Here's how the part is built. I have some questions about the finished solid (model axes, mm). A direction names the side the tool comes from. Coordinates: 2 decimals unless noted, no trailing zeros. Write each loop counter-clockwise with the first axis right and the second up, starting at its lowest first coordinate (ties: lowest second). Pieces come first, ordered by that corner, then holes.
Item 1: I want a section at C-C (x = 35.55). Please give me the cut outline in (y, z), and give its area (3 significant figures).
Item 2: I'm going to push flat-ended pins straight in: P1, Ø1.5, axis at x = 32, z = 6, coming from the -Y side; P2, Ø1.9, axis at x = 3.5, y = 3.5, coming from the -Z side; P3, Ø2, axis at y = -0.5, z = 2.5, coming from the -X side; P4, Ø3, axis at x = 24, y = -0.5, coming from the +Z side. Where does each tip first touch, or does it pass through?
Item 3: I want a section at D-D (y = -6.5). Please give me the cut outline in (x, z).
Item 4: I want a section at B-B (y = 10.65). Please give me the cut outline in (x, z).
Item 5: Please list where these lines run through material, in increasing order: line 1 (Y direction, x = 42.2, z = 0.8); line 2 (Y direction, x = 3.5, z = 1); line 3 (Z direction, x = 21, y = 5.5).
Item 6: I want a section at A-A (z = 2.5). Please give me the cut outline in (x, y).
Item 7: For faces 1 (the face through (25.85, 0, 2)), 2 (the face through (10, 11, 14.5)), 3 (the face through (24.35, -4.7, 2.48)), which set-ups out of +Z, -Z, +X, -X, +Y, -Y let a thin tool reach every point of the face, with its end or its side?
Autodesk Inventor part; units mm, degrees
ref_plane "YZ Plane" through (0, 0, 0) normal (1, 0, 0) x (0, 1, 0)
ref_plane "XZ Plane" through (0, 0, 0) normal (0, 1, 0) x (-1, 0, 0)
ref_plane "XY Plane" through (0, 0, 0) normal (0, 0, 1) x (1, 0, 0)
sketch "スケッチ1" plane through (0, 0, 0) normal (0, 0, 1) x (1, 0, 0)
  line L0 (0, 0) -> (45.7, 0)
  line L1 (45.7, 0) -> (45.7, 21.3)
  line L2 (45.7, 21.3) -> (0, 21.3)
  line L3 (0, 21.3) -> (0, 0)
  line L4 (45.7, 21.3) -> (42.2, 21.3) construction
  line L5 (42.2, 21.3) -> (42.2, 17.8) construction
  line L6 (42.2, 17.8) -> (45.7, 17.8) construction
  line L7 (45.7, 17.8) -> (45.7, 21.3) construction
  line L8 (0, 0) -> (3.5, 0) construction
  line L9 (3.5, 0) -> (3.5, 3.5) construction
  line L10 (3.5, 3.5) -> (0, 3.5) construction
  line L11 (0, 3.5) -> (0, 0) construction
  circle A0 centre (3.5, 3.5) radius 1.55
  circle A1 centre (42.2, 17.8) radius 1.55
  dimension "d0" = 45.7
  dimension "d1" = 21.3
  dimension "d2" = 3.5
  dimension "d3" = 3.5
  dimension "d4" = 3.5
  dimension "d5" = 3.5
  dimension "d6" = 3.1
  dimension "d7" = 3.1
extrude "押し出し1" add sketch "スケッチ1" along normal blind 1.5
sketch "スケッチ2" plane through (0, 0, 1.5) normal (0, 0, 1) x (1, 0, 0)
  line L0 (0, 21.3) -> (0, 0) construction
  line L1 (0, 10.65) -> (2, 10.65) construction
  line L2 (2, 10.65) -> (18.3, 10.65) construction
  line L3 (18.3, 10.65) -> (27.4, 10.65) construction
  line L4 (27.4, 10.65) -> (43.7, 10.65) construction
  line L5 (43.7, 10.65) -> (45.7, 10.65) construction
  circle A0 centre (10.15, 10.65) radius 8
  circle A1 centre (35.55, 10.65) radius 8
  dimension "d10" = 2
  dimension "d11" = 16.3
  dimension "d12" = 9.1
  dimension "d13" = 16.3
  dimension "d14" = 2
  dimension "d15" = 16
  dimension "d16" = 16
extrude "押し出し2" add sketch "スケッチ2" along normal blind 14
sketch "スケッチ3" plane through (10.15, 10.65, 15.5) normal (0, 0, 1) x (1, 0, 0)
  circle A0 centre (0, 0) radius 6.5
  circle A1 centre (25.4, 0) radius 8
  circle A2 centre (25.4, 0) radius 6.5
  point P0 (-10.15, -10.65)
  dimension "d19" = 13
  dimension "d20" = 13
extrude "押し出し3" cut sketch "スケッチ3" against normal blind 1 contours A0 | A2
sketch "スケッチ4" plane through (0, 0, 1.5) normal (0, 0, 1) x (1, 0, 0)
  line L0 (19.85, -1.25) -> (25.85, -1.25)
  line L1 (25.85, -1.25) -> (25.85, 1.25)
  line L2 (25.85, 1.25) -> (19.85, 1.25)
  line L3 (19.85, 1.25) -> (19.85, -1.25)
  line L4 (0, 0) -> (45.7, 0)
  line L5 (19.85, -1.25) -> (25.85, 1.25) construction
  line L6 (25.85, -1.25) -> (19.85, 1.25) construction
  point P0 (22.85, 0)
  dimension "d23" = 6
  dimension "d24" = 2.5
extrude "押し出し4" add sketch "スケッチ4" along normal blind 2
sketch "スケッチ5" plane through (19.85, -1.25, 1.5) normal (0, -1, 0) x (1, 0, 0)
  circle A0 centre (3, 1) radius 0.5
  line L0 (0, 0) -> (0, 2) construction
  line L1 (0, 1) -> (1, 1) construction
  line L2 (6, 0) -> (6, 2) construction
  line L3 (6, 1) -> (5, 1) construction
  circle A1 centre (1, 1) radius 0.5
  circle A2 centre (5, 1) radius 0.5
  point P0 (-19.85, -1.5)
  dimension "d27" = 1
  dimension "d28" = 1
  dimension "d29" = 1
  dimension "d30" = 1
  dimension "d31" = 1
extrude "押し出し5" add sketch "スケッチ5" along normal blind 7
properties part number "UltrasonicDistanceSencor"
Answer:
1. outline: (0, 0) - (21.3, 0) - (21.3, 1.5) - (18.65, 1.5) - (18.65, 15.5) - (17.15, 15.5) - (17.15, 14.5) - (4.15, 14.5) - (4.15, 15.5) - (2.65, 15.5) - (2.65, 1.5) - (0, 1.5) - close
1. area: 243 mm2
2. P1: stops at y = 3.16
2. P2: passes through
2. P3: stops at x = 19.85
2. P4: stops at z = 3.5
3. outline: circle Ø1 at (20.85, 2.5); circle Ø1 at (22.85, 2.5); circle Ø1 at (24.85, 2.5)
4. outline: (0, 0) - (45.7, 0) - (45.7, 1.5) - (43.55, 1.5) - (43.55, 15.5) - (42.05, 15.5) - (42.05, 14.5) - (29.05, 14.5) - (29.05, 15.5) - (27.55, 15.5) - (27.55, 1.5) - (18.15, 1.5) - (18.15, 15.5) - (16.65, 15.5) - (16.65, 14.5) - (3.65, 14.5) - (3.65, 15.5) - (2.15, 15.5) - (2.15, 1.5) - (0, 1.5) - close
5. line 1: y = 0 to 16.25, 19.35 to 21.3
5. line 2: y = 0 to 1.95, 5.05 to 21.3
5. line 3: z = 0 to 1.5
6. outline: circle Ø16 at (10.15, 10.65); (19.85, -1.25) - (20.35, -1.25) - (20.35, -8.25) - (21.35, -8.25) - (21.35, -1.25) - (22.35, -1.25) - (22.35, -8.25) - (23.35, -8.25) - (23.35, -1.25) - (24.35, -1.25) - (24.35, -8.25) - (25.35, -8.25) - (25.35, -1.25) - (25.85, -1.25) - (25.85, 1.25) - (19.85, 1.25) - close; circle Ø16 at (35.55, 10.65)
7. face 1: +Z, +X, +Y, -Y
7. face 2: +Z
7. face 3: -Y
